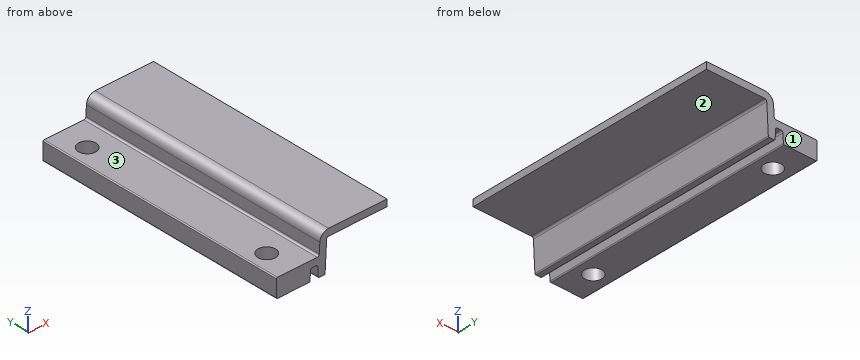
```python
from build123d import *

# Parameters (mm, degrees)
F1_DEPTH = 130
F3_D     = 9
F4_D     = 9


with BuildPart() as f1:
    # F0 (on Front) → F1 (new body)
    with BuildSketch(Plane.XZ):
        with BuildLine():
            Line((0, 8.5), (0, 0))
            ThreePointArc((0, 0), (0.146447, -0.353553), (0.5, -0.5))
            Line((0.5, -0.5), (16.760787, -0.5))
            ThreePointArc((16.760787, -0.5), (17.104964, -0.362687), (17.260102, -0.026168))
            Line((17.260102, -0.026168), (17.500051, 4.552336))
            ThreePointArc((17.500051, 4.552336), (17.810326, 5.225374), (18.49868, 5.5))
            Line((18.49868, 5.5), (20.261421, 5.5))
            ThreePointArc((20.261421, 5.5), (20.949776, 5.225374), (21.260051, 4.552336))
            Line((21.260051, 4.552336), (21.5, -0.026168))
            ThreePointArc((21.5, -0.026168), (21.655137, -0.362687), (21.999315, -0.5))
            Line((21.999315, -0.5), (24.500685, -0.5))
            ThreePointArc((24.500685, -0.5), (24.844863, -0.362687), (25, -0.026168))
            Line((25, -0.026168), (25.790231, 15.052336))
            ThreePointArc((25.790231, 15.052336), (26.100506, 15.725374), (26.78886, 16))
            Line((26.78886, 16), (56.78886, 16))
            Line((56.78886, 16), (56.78886, 19.5))
            Line((56.78886, 19.5), (26.78886, 19.5))
            ThreePointArc((26.78886, 19.5), (23.691265, 18.264185), (22.295028, 15.235512))
            Line((22.295028, 15.235512), (22.017903, 9.947664))
            ThreePointArc((22.017903, 9.947664), (21.707628, 9.274626), (21.019274, 9))
            Line((21.019274, 9), (0.5, 9))
            ThreePointArc((0.5, 9), (0.146447, 8.853553), (0, 8.5))
        make_face()
    extrude(amount=F1_DEPTH)

    # F3 (through all)
    with Locations(Plane.XY.offset(9)):
        with Locations((8.88, -15)):
            Hole(F3_D / 2)

    # F4 (through all)
    with Locations(Plane.XY.offset(9)):
        with Locations((8.88, -115)):
            Hole(F4_D / 2)


solid = f1.part
```
Geometry check sheet. Reference: the model listing, model coordinates, mm. Face numbers are marked on the shaded views. A direction names the side the tool comes from. Coordinates: 2 decimals unless noted, no trailing zeros. Order: outer loops, then holes, each group sorted by start corner. A loop starts at its lowest first (then second) coordinate and runs counter-clockwise, first axis right, second up. Notation, with made-up numbers: (-27, 43.25) - (27, 43.25) arc R19 ccw to (27, 76.25) - close; hole circle Ø6 at (42, 65). An arc over 180 degrees is marked (long way). Answer as a JSON object with one key per item and string values. Group by question number.
Item 1: Sectioned sample at A-A, the plane y = -115. Record the cut outline in (x, z).
Item 2: Scan lines: probe 1 along Y at (x, z) = (8.88, 3.25); probe 2 along Z at (x, y) = (47, -100); probe 3 along Z at (x, y) = (4, -18). Record each from-to range of solid material in increasing order.
Item 3: Sectioned sample at D-D, the plane y = -92. Record the cut outline in (x, z).
Item 4: Tool access check on the marked faces 1, 2 and 3. Record the directions out of +Z, -Z, +X, -X, +Y, -Y that give a thin tool (end or side, any length) a straight path to the whole face; none if there is none.
Item 5: Sectioned sample at B-B, the plane x = 8.88. Record the cut outline in (y, z), and give its area (3 significant figures).
Item 6: Sectioned sample at C-C, the plane z = 2. Record the cut outline in (x, y).
Item 7: Depth check by flat-ended pin: pin 1 Ø12 at (y, z) = (-56, 15.5) entering from -X; pin 2 Ø6 at (x, y) = (14.5, -37) entering from +Z; pin 3 Ø2 at (y, z) = (-83, 16.5) entering from -X. Enter the tip coordinate at first touch or a pass-through.
Resolved:
{
 "1": {"outline": "(0, 0) arc R0.5 ccw to (0.5, -0.5) - (4.38, -0.5) - (4.38, 9) - (0.5, 9) arc R0.5 ccw to (0, 8.5) - close; (13.38, -0.5) - (16.76, -0.5) arc R0.5 ccw to (17.26, -0.03) - (17.5, 4.55) arc R1 cw to (18.5, 5.5) - (20.26, 5.5) arc R1 cw to (21.26, 4.55) - (21.5, -0.03) arc R0.5 ccw to (22, -0.5) - (24.5, -0.5) arc R0.5 ccw to (25, -0.03) - (25.79, 15.05) arc R1 cw to (26.79, 16) - (56.79, 16) - (56.79, 19.5) - (26.79, 19.5) arc R4.5 ccw to (22.3, 15.24) - (22.02, 9.95) arc R1 cw to (21.02, 9) - (13.38, 9) - close"},
 "2": {"probe 1": "-130 to -119.5, -110.5 to -19.5, -10.5 to 0", "probe 2": "16 to 19.5", "probe 3": "-0.5 to 9"},
 "3": {"outline": "(0, 0) arc R0.5 ccw to (0.5, -0.5) - (16.76, -0.5) arc R0.5 ccw to (17.26, -0.03) - (17.5, 4.55) arc R1 cw to (18.5, 5.5) - (20.26, 5.5) arc R1 cw to (21.26, 4.55) - (21.5, -0.03) arc R0.5 ccw to (22, -0.5) - (24.5, -0.5) arc R0.5 ccw to (25, -0.03) - (25.79, 15.05) arc R1 cw to (26.79, 16) - (56.79, 16) - (56.79, 19.5) - (26.79, 19.5) arc R4.5 ccw to (22.3, 15.24) - (22.02, 9.95) arc R1 cw to (21.02, 9) - (0.5, 9) arc R0.5 ccw to (0, 8.5) - close"},
 "4": {"face 1": "+Z, -Z, +X, -X, +Y", "face 2": "-Z, +X, +Y, -Y", "face 3": "+Z, -X, +Y, -Y"},
 "5": {"outline": "(-130, -0.5) - (-119.5, -0.5) - (-119.5, 9) - (-130, 9) - close; (-110.5, -0.5) - (-19.5, -0.5) - (-19.5, 9) - (-110.5, 9) - close; (-10.5, -0.5) - (0, -0.5) - (0, 9) - (-10.5, 9) - close", "area": "1,060 mm^2"},
 "6": {"outline": "(0, -130) - (17.37, -130) - (17.37, 0) - (0, 0) - close; (21.39, -130) - (25.11, -130) - (25.11, 0) - (21.39, 0) - close; hole circle Ø9 at (8.88, -115); hole circle Ø9 at (8.88, -15)"},
 "7": {"pin 1": "x = 21.89", "pin 2": "z = 9", "pin 3": "x = 22.32"}
}
